```python
from build123d import *

# Parameters (mm, degrees)
CROQUIS1_W              = 19.05
CROQUIS1_H              = 12.7
SALIENTE_EXTRUIR1_DEPTH = 19.05
CROQUIS2_W              = 12.7
CROQUIS2_H              = 2.159
CORTAR_EXTRUIR1_DEPTH   = 23.235007389
CHAFL_N1_SIZE           = 3.048
CROQUIS9_R              = 5.1562
CORTAR_EXTRUIR4_DEPTH   = 6.35
CROQUIS17_R             = 3.2639
CORTAR_EXTRUIR5_DEPTH   = 25.797542721
REDONDEO1_START         = -9.525
REDONDEO1_DEPTH         = 19.05
CORTAR_EXTRUIR6_DEPTH   = 28.687044486
CORTAR_EXTRUIR7_DEPTH   = 28.687044486
CORTAR_EXTRUIR8_DEPTH   = 28.687044486
CORTAR_EXTRUIR9_DEPTH   = 28.687044486
CORTAR_EXTRUIR10_DEPTH  = 28.687044486
CORTAR_EXTRUIR11_DEPTH  = 28.687044486
CORTAR_EXTRUIR12_DEPTH  = 28.687044486
CORTAR_EXTRUIR13_DEPTH  = 28.687044486


with BuildPart() as part:
    # Croquis1 → Saliente-Extruir1 (new body)
    with BuildSketch(Plane(origin=(0, 0, 0), x_dir=(0, 0, -1), z_dir=(1, 0, 0))):
        with Locations((0, -0.034937632)):
            Rectangle(CROQUIS1_W, CROQUIS1_H)
    extrude(amount=SALIENTE_EXTRUIR1_DEPTH)

    # Croquis2 → Cortar-Extruir1 (cut, through all)
    with BuildSketch(Plane.ZY):
        with Locations((0, -5.305437632)):
            Rectangle(CROQUIS2_W, CROQUIS2_H)
    extrude(amount=-CORTAR_EXTRUIR1_DEPTH, mode=Mode.SUBTRACT)

    # Chaflán1
    chafl_n1_edges = [part.edges().sort_by_distance(p)[0] for p in [
        (19.05, -0.034937632, -9.525),
    ]]
    chamfer(chafl_n1_edges, length=CHAFL_N1_SIZE)

    # Croquis9 → Cortar-Extruir4 (cut)
    with BuildSketch(Plane(origin=(0, 6.315062368, 0), x_dir=(1, 0, 0), z_dir=(0, 1, 0))):
        with Locations(Location((6.35, 0, 0), (0, 0, 270))):
            Circle(CROQUIS9_R)
    extrude(amount=-CORTAR_EXTRUIR4_DEPTH, mode=Mode.SUBTRACT)

    # Croquis17 → Cortar-Extruir5 (cut, through all)
    with BuildSketch(Plane(origin=(0, 6.315062368, 0), x_dir=(1, 0, 0), z_dir=(0, 1, 0))):
        with Locations(Location((6.35, 0, 0), (0, 0, 270))):
            Circle(CROQUIS17_R)
    extrude(amount=-CORTAR_EXTRUIR5_DEPTH, mode=Mode.SUBTRACT)

    # Redondeo1: read off the stored shape, not the designer's step
    # Redondeo1 outline → Redondeo1 (cut)
    with BuildSketch(Plane.XY.offset(REDONDEO1_START)):
        with BuildLine():
            ThreePointArc((0, -3.336937632), (2.827005348, 3.48805702), (9.652, 6.315062368))
            Line((9.652, 6.315062368), (0, 6.315062368))
            Line((0, 6.315062368), (0, -3.336937632))
        make_face()
    extrude(amount=REDONDEO1_DEPTH, mode=Mode.SUBTRACT)

    # Croquis20 → Cortar-Extruir6 (cut, through all)
    with BuildSketch(Plane.XY.offset(9.525)):
        Polygon((19.05, -6.384937632), (19.05, -4.860937632), (17.517257595, -4.860937632), align=None)
    extrude(amount=-CORTAR_EXTRUIR6_DEPTH, mode=Mode.SUBTRACT)

    # Croquis21 → Cortar-Extruir7 (cut, through all)
    with BuildSketch(Plane.XY.offset(9.525)):
        Polygon((19.05, -4.860937632), (19.05, -3.336937632), (17.526, -3.336937632), align=None)
    extrude(amount=-CORTAR_EXTRUIR7_DEPTH, mode=Mode.SUBTRACT)

    # Croquis22 → Cortar-Extruir8 (cut, through all)
    with BuildSketch(Plane.XY.offset(9.525)):
        Polygon((19.05, -3.336937632), (19.05, -1.812937632), (17.526, -1.812937632), align=None)
    extrude(amount=-CORTAR_EXTRUIR8_DEPTH, mode=Mode.SUBTRACT)

    # Croquis23 → Cortar-Extruir9 (cut, through all)
    with BuildSketch(Plane.XY.offset(9.525)):
        Polygon((19.05, -1.812937632), (19.05, -0.288937632), (17.526, -0.288937632), align=None)
    extrude(amount=-CORTAR_EXTRUIR9_DEPTH, mode=Mode.SUBTRACT)

    # Croquis24 → Cortar-Extruir10 (cut, through all)
    with BuildSketch(Plane.XY.offset(9.525)):
        Polygon((19.05, -0.288937632), (19.05, 1.235062368), (17.526, 1.235062368), align=None)
    extrude(amount=-CORTAR_EXTRUIR10_DEPTH, mode=Mode.SUBTRACT)

    # Croquis25 → Cortar-Extruir11 (cut, through all)
    with BuildSketch(Plane.XY.offset(9.525)):
        Polygon((19.05, 1.235062368), (19.05, 2.759062368), (17.526, 2.759062368), align=None)
    extrude(amount=-CORTAR_EXTRUIR11_DEPTH, mode=Mode.SUBTRACT)

    # Croquis26 → Cortar-Extruir12 (cut, through all)
    with BuildSketch(Plane.XY.offset(9.525)):
        Polygon((19.05, 2.759062368), (19.05, 4.283062368), (17.526, 4.283062368), align=None)
    extrude(amount=-CORTAR_EXTRUIR12_DEPTH, mode=Mode.SUBTRACT)

    # Croquis27 → Cortar-Extruir13 (cut, through all)
    with BuildSketch(Plane.XY.offset(9.525)):
        Polygon((19.05, 4.283062368), (16.672562903, 6.315062368), (19.05, 6.315062368), align=None)
    extrude(amount=-CORTAR_EXTRUIR13_DEPTH, mode=Mode.SUBTRACT)


solid = part.part
```
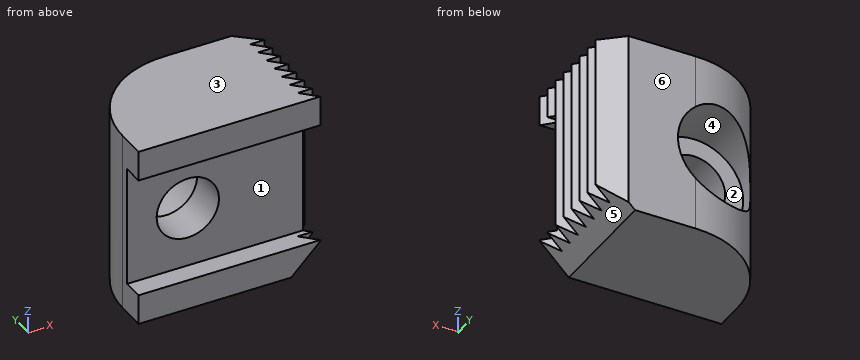
Check sheet for the modelled part. Datum: model origin and axes. Units: mm. Face numbers are marked on the shaded views. A direction names the side the tool comes from. Give positions to 0.01 mm unless a question says otherwise; leave off trailing zeros. Write each loop counter-clockwise with the first axis right and the second up, starting at its lowest first coordinate (ties: lowest second). Pieces come first, ordered by that corner, then holes.
Item 1: Scan lines: L1, parallel to Z at x = 6.35, y = 2 (3 decimals); L2, parallel to Z at x = 15.75, y = -4.5 (3 decimals); L3, parallel to Y at x = 15, z = 2.25. Record each from-to range of solid material in increasing order.
Item 2: Cross-section at D-D (y = 1.75). Enter the section's corners in (x, z) (3 decimals).
Item 3: Draft check along Z on the marked faces 4, 5 and 6. Enter one of: released by +Z, released by -Z, zero draft, split by the parting line, or undercut.
Item 4: Cross-section at A-A (z = 5.5). Enter the section's corners in (x, y) (3 decimals).
Item 5: Cross-section at C-C (z = -1.25). Enter the section's corners in (x, y) (3 decimals).
Item 6: Gauge pin test, flat ends, axial feed: pin 1 (1.7 mm diameter, centred on x = 18.5, z = 0.5, fed in from -Y); pin 2 (6 mm diameter, centred on y = 5, z = 5, fed in from -X); pin 3 (1 mm diameter, centred on y = -0.5, z = -6.5, fed in from -X). Record the tip position at first contact, or that the pin passes through.
Item 7: Cross-section at B-B (x = 15). Enter the section's corners in (y, z) (3 decimals), and give its area (3 significant figures).
Item 8: Access from +Z, -Z, +X, -X, +Y, -Y to the whole of each face (thin tool, end or side, straight path). Record for the marked faces 1, 2 and 3.
Report:
1. L1: z = -9.525 to -5.156, 5.156 to 9.525
1. L2: z = -9.525 to -6.35, 6.35 to 9.525
1. L3: y = -4.23 to 6.32
2. outline: (1.449, -9.525) - (16.002, -9.525) - (18.535, -6.992) - (18.535, 9.525) - (1.449, 9.525) - (1.449, 1.603) arc R5.156 cw (long way) to (1.449, -1.603) - close
3. face 4: undercut
3. face 5: released by -Z
3. face 6: zero draft
4. outline: (0, -4.226) - (18.415, -4.226) - (17.526, -3.337) - (19.05, -3.337) - (17.526, -1.813) - (19.05, -1.813) - (17.526, -0.289) - (19.05, -0.289) - (17.526, 1.235) - (19.05, 1.235) - (17.526, 2.759) - (19.05, 2.759) - (17.526, 4.283) - (19.05, 4.283) - (16.673, 6.315) - (9.652, 6.315) arc R9.652 ccw to (0, -3.337) - close
5. outline: (0, -4.226) - (3.335, -4.226) - (3.335, -0.035) - (1.348, -0.035) - (1.348, 1.582) arc R9.652 ccw to (0, -3.337) - close; (9.365, -4.226) - (18.415, -4.226) - (17.526, -3.337) - (19.05, -3.337) - (17.526, -1.813) - (19.05, -1.813) - (17.526, -0.289) - (19.05, -0.289) - (17.526, 1.235) - (19.05, 1.235) - (17.526, 2.759) - (19.05, 2.759) - (17.526, 4.283) - (19.05, 4.283) - (16.673, 6.315) - (11.352, 6.315) - (11.352, -0.035) - (9.365, -0.035) - close
6. pin 1: stops at y = -4.23
6. pin 2: stops at x = 1.61
6. pin 3: stops at x = 0.29
7. outline: (-6.385, -9.525) - (6.315, -9.525) - (6.315, 9.525) - (-6.385, 9.525) - (-6.385, 6.35) - (-4.226, 6.35) - (-4.226, -6.35) - (-6.385, -6.35) - close
7. area: 215 mm2
8. face 1: +X, -X, -Y
8. face 2: +Y
8. face 3: +Z, +X, -X, +Y, -Y
